Read the model definition and answer for the solid it produces. Units are mm, in the model's axes. A direction names the side the tool comes from. Round coordinates to 2 decimals unless told otherwise and drop trailing zeros. Write each loop counter-clockwise with the first axis right and the second up, starting at its lowest first coordinate (ties: lowest second). Pieces come first, ordered by that corner, then holes.
from build123d import *

# Parameters (mm, degrees)
SKETCH_1_W          = 9.5
SKETCH_1_H          = 9.5
EXTRUDE_1_DEPTH     = 4
SKETCH_1_4_W        = 1.5
SKETCH_1_4_H        = 8
EXTRUDE_2_DEPTH     = 1
SKETCH_1_5_W        = 1
SKETCH_1_5_H        = 0.3
SKETCH_1_5_W_2      = 0.3
SKETCH_1_5_H_2      = 1
CUT_EXTRUDE_1_DEPTH = 0.2


with BuildPart() as part:
    # 草图1 → 凸台-拉伸1 (new body)
    with BuildSketch(Plane(origin=(0, 0, 0), x_dir=(0, 0, -1), z_dir=(1, 0, 0))):
        with Locations((4.75, 4.75)):
            Rectangle(SKETCH_1_W, SKETCH_1_H)
    extrude(amount=EXTRUDE_1_DEPTH)

    # 草图1<4> → 凸台-拉伸2 (add)
    with BuildSketch(Plane(origin=(0, 0, 0), x_dir=(0, 0, -1), z_dir=(1, 0, 0))):
        with Locations((6.583333333, 5.5)):
            Rectangle(SKETCH_1_4_W, SKETCH_1_4_H)
        with Locations((2.916666667, 5.5)):
            Rectangle(SKETCH_1_4_W, SKETCH_1_4_H)
    extrude(amount=-EXTRUDE_2_DEPTH)

    # 草图1<5> → 切除-拉伸1 (cut)
    with BuildSketch(Plane(origin=(0, 0, 0), x_dir=(0, 0, -1), z_dir=(1, 0, 0))):
        with Locations((6.583333333, 0.75)):
            Rectangle(SKETCH_1_5_W, SKETCH_1_5_H)
        with Locations((6.583333333, 0.75)):
            Rectangle(SKETCH_1_5_W_2, SKETCH_1_5_H_2)
        with Locations((2.916666667, 0.75)):
            Rectangle(SKETCH_1_5_W, SKETCH_1_5_H)
    extrude(amount=CUT_EXTRUDE_1_DEPTH, mode=Mode.SUBTRACT)


solid = part.part
Q1. Section B-B (z = -6.25) is taken. Determine the outline of the cut face in (x, y), then the cut area to 3 significant figures.
Verdict:
outline: (-1, 1.5) - (0, 1.5) - (0, 0.9) - (0.2, 0.9) - (0.2, 0.6) - (0, 0.6) - (0, 0) - (4, 0) - (4, 9.5) - (-1, 9.5) - close
area: 45.9 mm2
Q2. Determine the mould class of faces 1 (the flat face through (-0.5, 5.4, -3.667)), 2 (the flat face through (2, 5, -9.5)), 3 (the flat face through (0, 5, -5)), 4 (the flat face through (-0.5, 1.5, -6.6)) for opening direction Z: pulls with the +Z half, pulls with the -Z half, needs draft (parallel to the pull), parting line crosses it, or undercut.
Verdict:
face 1: undercut
face 2: pulls with the -Z half
face 3: undercut
face 4: needs draft
Q3. Flat-ended cylindrical pins translate along their axes: pin 1 Ø0.5 at (y, z) = (1, -7) entering from -X; pin 2 Ø0.8 at (x, z) = (-0.5, -6.5) entering from -Y. Find the tip coordinate at first contact, or state that the pin passes through.
Verdict:
pin 1: stops at x = 0
pin 2: stops at y = 1.5
Q4. Section A-A (y = 2.75) is taken. Determine the outline of the cut face in (x, z), then the cut area to 3 significant figures.
Verdict:
outline: (-1, -7.33) - (0, -7.33) - (0, -9.5) - (4, -9.5) - (4, 0) - (0, 0) - (0, -2.17) - (-1, -2.17) - (-1, -3.67) - (0, -3.67) - (0, -5.83) - (-1, -5.83) - close
area: 41.0 mm2
Q5. Section C-C (z = -7.75) is taken. Determine the outline of the cut face in (x, y).
Verdict:
outline: (0, 0) - (4, 0) - (4, 9.5) - (0, 9.5) - close
Q6. Which of the six approach directions +Z, -Z, +X, -X, +Y, -Y give full straight-line access (tool end or side, diameter ignored) to faces 5 (the flat face through (-0.5, 1.5, -2.9)), 6 (the flat face through (-0.5, 5.4, -2.167)), 7 (the flat face through (-0.5, 5.4, -7.333)), 8 (the flat face through (-0.5, 5.4, -5.833)), 9 (the flat face through (2, 0, -5))?
Verdict:
face 5: +Z, -Z, -X, -Y
face 6: +Z, -X, +Y, -Y
face 7: -Z, -X, +Y, -Y
face 8: -X, +Y, -Y
face 9: +Z, -Z, +X, -X, -Y
Q7. Straight lines are drawn through the part: probe 1 along Z at (x, y) = (-0.45, 6); probe 2 along X at (y, z) = (7.75, -8). For each, find the intervals that lie inside material, in ascending order.
Verdict:
probe 1: z = -7.33 to -5.83, -3.67 to -2.17
probe 2: x = 0 to 4
